CAD build for the part. Positions are in the model's coordinates, mm. Face numbers are marked on the shaded views. A direction names the side the tool comes from. Give positions to 0.01 mm unless a question says otherwise; leave off trailing zeros. Write each loop counter-clockwise with the first axis right and the second up, starting at its lowest first coordinate (ties: lowest second). Pieces come first, ordered by that corner, then holes. Notation, with made-up numbers: (55.5, 27.25) - (99.5, 27.25) arc R29 cw to (99.5, 55.25) - close; hole circle Ø10 at (58.5, 4.5). An arc over 180 degrees is marked (long way). Answer as a JSON object with one key per item and string values.
from build123d import *

# Parameters (mm, degrees)
F0_R     = 7.5
F1_DEPTH = 7.5
F2_DEPTH = 3.5


with BuildPart() as f1:
    # F0 (on Top) → F1 (new body, symmetric)
    with BuildSketch(Plane.XY):
        with BuildLine():
            Line((32.020504, 8.144187), (12.020504, 8.144187))
            Line((12.020504, 8.144187), (12.020504, -10.855813))
            Line((12.020504, -10.855813), (32.020504, -10.855813))
            ThreePointArc((32.020504, -10.855813), (41.520504, -1.355813), (32.020504, 8.144187))
        make_face()
        with Locations((32.020504, -1.355813)):
            Circle(F0_R, mode=Mode.SUBTRACT)
        with BuildLine():
            Line((32.020504, 13.644187), (12.020504, 13.644187))
            Line((12.020504, 13.644187), (12.020504, 8.144187))
            Line((12.020504, 8.144187), (32.020504, 8.144187))
            ThreePointArc((32.020504, 8.144187), (41.520504, -1.355813), (32.020504, -10.855813))
            Line((32.020504, -10.855813), (12.020504, -10.855813))
            Line((12.020504, -10.855813), (12.020504, -16.355813))
            Line((12.020504, -16.355813), (32.020504, -16.355813))
            ThreePointArc((32.020504, -16.355813), (47.020504, -1.355813), (32.020504, 13.644187))
        make_face()
    extrude(amount=F1_DEPTH, both=True)

    # F0 (on Top) → F2 (cut, symmetric)
    with BuildSketch(Plane.XY):
        with BuildLine():
            Line((32.020504, 13.644187), (12.020504, 13.644187))
            Line((12.020504, 13.644187), (12.020504, 8.144187))
            Line((12.020504, 8.144187), (32.020504, 8.144187))
            ThreePointArc((32.020504, 8.144187), (41.520504, -1.355813), (32.020504, -10.855813))
            Line((32.020504, -10.855813), (12.020504, -10.855813))
            Line((12.020504, -10.855813), (12.020504, -16.355813))
            Line((12.020504, -16.355813), (32.020504, -16.355813))
            ThreePointArc((32.020504, -16.355813), (47.020504, -1.355813), (32.020504, 13.644187))
        make_face()
    extrude(amount=F2_DEPTH, both=True, mode=Mode.SUBTRACT)


solid = f1.part
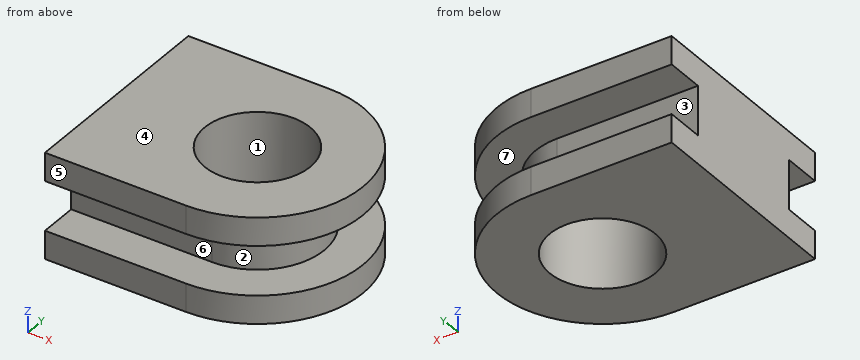
Item 1: Flat gauge pins, fed straight in: P1, Ø4, axis at x = 16.5, z = 0, coming from the +Y side; P2, Ø2, axis at y = -12.5, z = 3, coming from the +X side; P3, Ø2, axis at x = 42, z = 5.5, coming from the -Y side. Where does each tip first touch, or does it go through?
Entries:
{"P1": "y = 8.14", "P2": "x = 42.95", "P3": "y = -13.37"}
Item 2: Mould opens along Z. For the marked faces 4, 5, 6 and 7 say: +Z half, -Z half, draft (parallel to the pull), parting line (faces both ways), or undercut.
Entries:
{"face 4": "+Z half", "face 5": "draft", "face 6": "undercut", "face 7": "undercut"}
Item 3: Cut at B-B (y = 5). Give the cut face in (x, z).
Entries:
{"outline": "(12.02, -7.5) - (28.04, -7.5) - (28.04, 7.5) - (12.02, 7.5) - close; (36, -7.5) - (45.61, -7.5) - (45.61, -3.5) - (39.08, -3.5) - (39.08, 3.5) - (45.61, 3.5) - (45.61, 7.5) - (36, 7.5) - close"}
Item 4: Cut at C-C (z = -4.75). Give the cut face in (x, y), and give its area (3 significant figures).
Entries:
{"outline": "(12.02, -16.36) - (32.02, -16.36) arc R15 ccw to (32.02, 13.64) - (12.02, 13.64) - close; hole circle Ø15 at (32.02, -1.36)", "area": "777 mm2"}
Item 5: Which spindle directions (+Z, -Z, +X, -X, +Y, -Y) get a long thin tool onto all of the face, cutting with end or side? Do the marked faces 1, 2 and 3. Say none if no direction does.
Entries:
{"face 1": "+Z, -Z", "face 2": "+X", "face 3": "+X, -X, +Y"}
Item 6: Probe line 1 (X direction, y = -1.5, z = -3.75); line 2 (Z direction, x = 28, y = -14.75); line 3 (X direction, y = 3.25, z = 6). List the from-to ranges inside material, lowest first. Write a range as from..to.
Entries:
{"line 1": "12.02..24.52, 39.52..47.02", "line 2": "-7.5..-3.5, 3.5..7.5", "line 3": "12.02..26.1, 37.94..46.3"}
Item 7: Cut at D-D (x = 17). Give the cut face in (y, z), and give its area (3 significant figures).
Entries:
{"outline": "(-16.36, -7.5) - (13.64, -7.5) - (13.64, -3.5) - (8.14, -3.5) - (8.14, 3.5) - (13.64, 3.5) - (13.64, 7.5) - (-16.36, 7.5) - (-16.36, 3.5) - (-10.86, 3.5) - (-10.86, -3.5) - (-16.36, -3.5) - close", "area": "373 mm2"}
Item 8: Cut at A-A (x = 44). Give the cut face in (y, z), and give its area (3 significant figures).
Entries:
{"outline": "(-10.38, -7.5) - (7.67, -7.5) - (7.67, -3.5) - (-10.38, -3.5) - close; (-10.38, 3.5) - (7.67, 3.5) - (7.67, 7.5) - (-10.38, 7.5) - close", "area": "144 mm2"}
